```python
from build123d import *

# Parameters (mm, degrees)
SKETCH_1_W             = 40
SKETCH_1_H             = 40
EXTRUDE_1_DEPTH        = 60
SKETCH_2_R             = 15.1
CUT_EXTRUDE_1_DEPTH    = 50
SKETCH_3_W             = 40
SKETCH_3_H             = 30
SKETCH_3_R             = 1.5
EXTRUDE_2_DEPTH        = 5
FILLET_1_R             = 5
SKETCH_4_R             = 1.5
CUT_EXTRUDE_2_DEPTH    = 75.833147735
PATTERN_LINEAR_1_COUNT = 2
PATTERN_LINEAR_1_PITCH = 20


with BuildPart() as part:
    # 草圖1 → 填料-伸長1 (new body)
    with BuildSketch(Plane(origin=(0, 0, 0), x_dir=(1, 0, 0), z_dir=(0, 1, 0))):
        Rectangle(SKETCH_1_W, SKETCH_1_H)
    extrude(amount=EXTRUDE_1_DEPTH)

    # 草圖2 → 除料-伸長1 (cut)
    with BuildSketch(Plane(origin=(0, 60, 0), x_dir=(1, 0, 0), z_dir=(0, 1, 0))):
        with Locations(Location((0, 0, 0), (0, 0, 270))):
            Circle(SKETCH_2_R)
    extrude(amount=-CUT_EXTRUDE_1_DEPTH, mode=Mode.SUBTRACT)

    # 草圖3 → 填料-伸長2 (add)
    with BuildSketch(Plane.XY.offset(20)):
        with Locations((0, -15)):
            Rectangle(SKETCH_3_W, SKETCH_3_H)
        with Locations((-12, -8)):
            Circle(SKETCH_3_R, mode=Mode.SUBTRACT)
        with Locations((-12, -22)):
            Circle(SKETCH_3_R, mode=Mode.SUBTRACT)
        with Locations(Location((12, -22, 0), (0, 0, 180))):
            Circle(SKETCH_3_R, mode=Mode.SUBTRACT)
        with Locations(Location((12, -8, 0), (0, 0, 180))):
            Circle(SKETCH_3_R, mode=Mode.SUBTRACT)
    extrude(amount=-EXTRUDE_2_DEPTH)

    # 圓角1
    fillet_1_edges = [part.edges().sort_by_distance(p)[0] for p in [
        (-20, -30, 17.5),
        (20, -30, 17.5),
    ]]
    fillet(fillet_1_edges, radius=FILLET_1_R)

    # 草圖4 → 除料-伸長2 (cut, through all)
    with BuildSketch(Plane(origin=(0, 0, -20), x_dir=(-1, 0, 0), z_dir=(0, 0, -1))):
        with Locations((0, 20)):
            Circle(SKETCH_4_R)
    cut_extrude_2 = extrude(amount=-CUT_EXTRUDE_2_DEPTH, mode=Mode.SUBTRACT)

    # 直線複製排列1: 除料-伸長2 ×2
    with Locations(*[(0, i * PATTERN_LINEAR_1_PITCH, 0) for i in range(1, PATTERN_LINEAR_1_COUNT)]):
        add(cut_extrude_2, mode=Mode.SUBTRACT)


solid = part.part
```
Could you check a few things on this model? Use its own coordinates, in mm. A direction names the side the tool comes from. Coordinates: 2 decimals unless noted, no trailing zeros. Write each loop counter-clockwise with the first axis right and the second up, starting at its lowest first coordinate (ties: lowest second). Pieces come first, ordered by that corner, then holes. Notation, with made-up numbers: M -7.75,7 L 10.25,7 A32 ccw 10.25,35 Z; hole C 42.5,76 d3. An arc over 180 degrees is marked long. Answer as CSV lines item,"result". Start each with the question number.
1) For P1, Ø1.8, axis at x = 0, y = 20, coming from the -Z side; P2, Ø15, axis at x = 4, z = -4, coming from the +Y side; P3, Ø1, axis at x = 13.5, z = -14, coming from the -Y side; P4, Ø9, axis at x = -9.5, y = -21, coming from the -Z side, each with a flat end and sliding along its axis, tell me the tip position at first contact or that it passes through.
2) I want a section at D-D, the plane x = 12. Please give me the cut outline in (y, z), and give its area (3 significant figures).
3) We'd pull the mould along X, two halves only. Please class faces 4 (the cylindrical face through (-19, -28, 17)), 5 (the cylindrical face through (0.325, 38.536, -17.547)), 6 (the flat face through (0, 10, 0)), 7 (the flat face through (0, 16, 20)): +X half, -X half, draft (parallel to the pull), parting line (faces both ways), or undercut.
4) Please list where these lines run through material, in increasing order: line 1 (Y direction, x = 0, z = -18.8); line 2 (Y direction, x = 0, z = 17.4); line 3 (X direction, y = 40, z = -17.95). Write a range as from..to.
5) For faces 1 (the flat face through (-20, 26, 0)), 2 (the cylindrical face through (-5.78, 35.35, 13.95)), 3 (the flat face through (0, -15, 15)), which set-ups out of +Z, -Z, +X, -X, +Y, -Y let a thin tool reach every point of the face, with its end or its side?
6) I want a section at C-C, the plane z = 1.5. Please give me the cut outline in (x, y).
7) I want a section at B-B, the plane x = 0. Please give me the cut outline in (y, z).
8) I want a section at A-A, the plane y = 20. Please give me the cut outline in (x, z), and give its area (3 significant figures).
Data:
1,P1,"passes through"
1,P2,"stops at y = 10"
1,P3,"stops at y = 0"
1,P4,"stops at z = 15"
2,outline,"M -30,15 L -23.5,15 L -23.5,20 L -30,20 Z; M -20.5,15 L -9.5,15 L -9.5,20 L -20.5,20 Z; M -6.5,15 L 0,15 L 0,-20 L 60,-20 L 60,-9.17 L 10,-9.17 L 10,9.17 L 60,9.17 L 60,20 L -6.5,20 Z"
2,area,"1,600 mm^2"
3,face 4,"-X half"
3,face 5,"undercut"
3,face 6,"undercut"
3,face 7,"draft"
4,line 1,"y = 0..18.5, 21.5..38.5, 41.5..60"
4,line 2,"y = -30..18.5, 21.5..38.5, 41.5..60"
4,line 3,"x = -20..-1.5, 1.5..20"
5,face 1,"+Z, -Z, -X, +Y, -Y"
5,face 2,"+Y"
5,face 3,"-Z, +X, -X, -Y"
6,outline,"M -20,0 L 20,0 L 20,60 L 15.03,60 L 15.03,10 L -15.03,10 L -15.03,60 L -20,60 Z"
7,outline,"M -30,15 L 0,15 L 0,-20 L 18.5,-20 L 18.5,-15.1 L 10,-15.1 L 10,15.1 L 18.5,15.1 L 18.5,20 L -30,20 Z; M 21.5,-20 L 38.5,-20 L 38.5,-15.1 L 21.5,-15.1 Z; M 21.5,15.1 L 38.5,15.1 L 38.5,20 L 21.5,20 Z; M 41.5,-20 L 60,-20 L 60,-15.1 L 41.5,-15.1 Z; M 41.5,15.1 L 60,15.1 L 60,20 L 41.5,20 Z"
8,outline,"M -20,-20 L -1.5,-20 L -1.5,-15.03 A15.1 cw -1.5,15.03 L -1.5,20 L -20,20 Z; M 1.5,-20 L 20,-20 L 20,20 L 1.5,20 L 1.5,15.03 A15.1 cw 1.5,-15.03 Z"
8,area,"854 mm^2"
